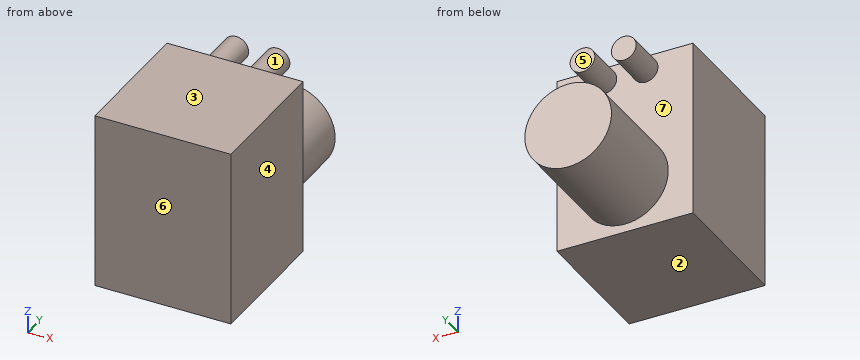
from build123d import *

# Parameters (mm, degrees)
SKETCH_1_W      = 66
SKETCH_1_H      = 66
EXTRUDE_1_DEPTH = 86
SKETCH_2_R      = 21
EXTRUDE_2_DEPTH = 52
SKETCH_3_R      = 6
EXTRUDE_3_DEPTH = 20


with BuildPart() as part:
    # 草图1 → 凸台-拉伸1 (new body)
    with BuildSketch(Plane.XY):
        Rectangle(SKETCH_1_W, SKETCH_1_H)
    extrude(amount=EXTRUDE_1_DEPTH)

    # 草图2 → 凸台-拉伸2 (add)
    with BuildSketch(Plane(origin=(0, 33, 0), x_dir=(1, 0, 0), z_dir=(0, 1, 0))):
        with Locations((0, -25)):
            Circle(SKETCH_2_R)
    extrude(amount=EXTRUDE_2_DEPTH)

    # 草图3 → 凸台-拉伸3 (add)
    with BuildSketch(Plane(origin=(0, 33, 0), x_dir=(1, 0, 0), z_dir=(0, 1, 0))):
        with Locations((-10, -79)):
            Circle(SKETCH_3_R)
        with Locations((10, -79)):
            Circle(SKETCH_3_R)
    extrude(amount=EXTRUDE_3_DEPTH)


solid = part.part
Part model, mm, in its own coordinate system. Face numbers are marked on the shaded views. A direction names the side the tool comes from. Give positions to 0.01 mm unless a question says otherwise; leave off trailing zeros. Write each loop counter-clockwise with the first axis right and the second up, starting at its lowest first coordinate (ties: lowest second). Pieces come first, ordered by that corner, then holes.
1) Cut at D-D on z = 25. Write the cut outline in (x, y).
Resolved:
outline: (-33, -33) - (33, -33) - (33, 33) - (21, 33) - (21, 85) - (-21, 85) - (-21, 33) - (-33, 33) - close
2) Cut at C-C on y = 50.5. Write the cut outline in (x, z), then the cut area to 3 significant figures.
Resolved:
outline: circle Ø42 at (0, 25); circle Ø12 at (-10, 79); circle Ø12 at (10, 79)
area: 1,610 mm2
3) Cut at A-A on z = 79. Write the cut outline in (x, y), then the cut area to 3 significant figures.
Resolved:
outline: (-33, -33) - (33, -33) - (33, 33) - (16, 33) - (16, 53) - (4, 53) - (4, 33) - (-4, 33) - (-4, 53) - (-16, 53) - (-16, 33) - (-33, 33) - close
area: 4,840 mm2
4) Which spindle directions (+Z, -Z, +X, -X, +Y, -Y) get a long thin tool onto all of the face, cutting with end or side? Do the marked faces 5, 6 and 7. Say none if no direction does.
Resolved:
face 5: +Z, +X, -X, +Y
face 6: +Z, -Z, +X, -X, -Y
face 7: +Y
5) Probe L1, parallel to Y at x = 25.5, z = 10; L2, parallel to Y at x = -9, z = 77.5; L3, parallel to Z at x = -9.5, y = 38. List the from-to ranges inside material, lowest first.
Resolved:
L1: y = -33 to 33
L2: y = -33 to 53
L3: z = 6.27 to 43.73, 73.02 to 84.98
6) Pin check, flat tips, straight feed: pin 1 (13 mm diameter, centred on x = -10, z = 76, fed in from +Y); pin 2 (10 mm diameter, centred on y = 51.5, z = 19.5, fed in from +X); pin 3 (12 mm diameter, centred on x = -17, z = 50, fed in from +Y). Stop position of each tip, or through.
Resolved:
pin 1: stops at y = 53
pin 2: stops at x = 20.99
pin 3: stops at y = 33
7) Two-plate mould, pull along Z, no slides. Class the marked faces 1, 2, 3 and 4: released by +Z, released by -Z, zero draft, split by the parting line, or undercut.
Resolved:
face 1: undercut
face 2: released by -Z
face 3: released by +Z
face 4: zero draft
8) Cut at B-B on x = 0. Write the cut outline in (y, z), then the cut area to 3 significant figures.
Resolved:
outline: (-33, 0) - (33, 0) - (33, 4) - (85, 4) - (85, 46) - (33, 46) - (33, 86) - (-33, 86) - close
area: 7,860 mm2
